Check sheet for the modelled part. Datum: model origin and axes. Units: mm. Give positions to 0.01 mm unless a question says otherwise; leave off trailing zeros. Order: outer loops, then holes, each group sorted by start corner. A loop starts at its lowest first (then second) coordinate and runs counter-clockwise, first axis right, second up. Notation, with made-up numbers: M -26,-38.75 L -11,-38.75 A24 ccw -11,-4.75 Z; hole C -1.5,9 d11. An arc over 180 degrees is marked long. Return JSON: item names as keys, results as strings. Group by question number.
from build123d import *

# Parameters (mm, degrees)
SKETCH1_R           = 9.54
BOSS_EXTRUDE1_DEPTH = 300
BOSS_EXTRUDE2_START = -60
BOSS_EXTRUDE2_DEPTH = 60


with BuildPart() as part:
    # Sketch1 → Boss-Extrude1 (new body)
    with BuildSketch(Plane(origin=(0, 0, 0), x_dir=(1, 0, 0), z_dir=(0, 1, 0))):
        with Locations(Location((0, 0, 0), (0, 0, 270))):
            Circle(SKETCH1_R)
    extrude(amount=BOSS_EXTRUDE1_DEPTH)

    # Sketch2 → Boss-Extrude2 (add)
    with BuildSketch(Plane(origin=(0, 300, 0), x_dir=(1, 0, 0), z_dir=(0, 1, 0)).offset(BOSS_EXTRUDE2_START)):
        with BuildLine():
            Line((-2.4, 9.233179301), (-2.4, 11.87))
            Line((-2.4, 11.87), (2.4, 11.87))
            Line((2.4, 11.87), (2.4, 9.233179301))
            ThreePointArc((2.4, 9.233179301), (0, 9.54), (-2.4, 9.233179301))
        make_face()
    extrude(amount=BOSS_EXTRUDE2_DEPTH)


solid = part.part
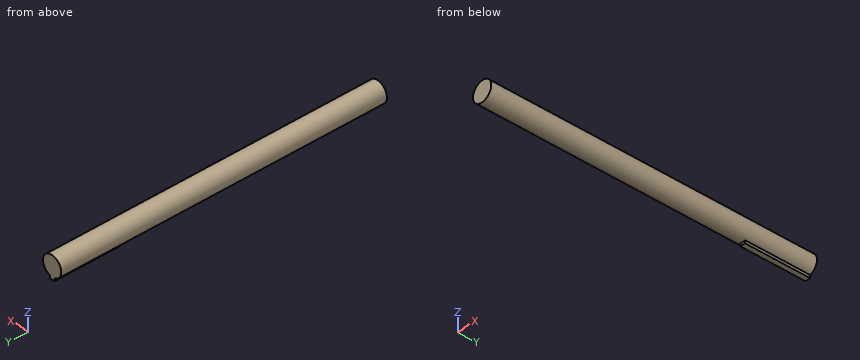
1) Sectioned sample at A-A on y = 96. Record the boundary of the cut face in (x, z).
2) Sectioned sample at C-C on x = -5.5. Record the boundary of the cut face in (y, z), then the cut area to 3 significant figures.
3) Material ranges on line 1 along Z through (x, y) = (0.5, 249); line 2 along Z through (x, y) = (-0.25, 142.5); line 3 along X through (y, z) = (61, 1), recorded low to high.
4) Depth check by flat-ended pin: P1, Ø1.5, axis at x = -4.5, y = 35, coming from the +Z side; P2, Ø6, axis at y = 184, z = -9, coming from the -X side; P3, Ø2, axis at y = 283.5, z = -11, coming from the +X side. Enter the tip coordinate at first touch or a pass-through.
5) Sectioned sample at B-B on z = 5.5. Record the boundary of the cut face in (x, y), then the cut area to 3 significant figures.
Reply:
{
 "1": {"outline": "C 0,0 d19.08"},
 "2": {"outline": "M 0,-7.79 L 300,-7.79 L 300,7.79 L 0,7.79 Z", "area": "4,680 mm^2"},
 "3": {"line 1": "-11.87 to 9.53", "line 2": "-9.54 to 9.54", "line 3": "-9.49 to 9.49"},
 "4": {"P1": "z = 8.77", "P2": "x = -7.42", "P3": "x = 2.4"},
 "5": {"outline": "M -7.79,0 L 7.79,0 L 7.79,300 L -7.79,300 Z", "area": "4,680 mm^2"}
}
